Verification items for the finished model (mm, model axes). A direction names the side the tool comes from. Give positions to 0.01 mm unless a question says otherwise; leave off trailing zeros. Write each loop counter-clockwise with the first axis right and the second up, starting at its lowest first coordinate (ties: lowest second). Pieces come first, ordered by that corner, then holes.
from build123d import *

# Parameters (mm, degrees)
SKETCH_5_W          = 30.974653289
SKETCH_5_H          = 53.868777402
SKETCH_5_W_2        = 27.381586342
SKETCH_5_H_2        = 50.41539456
EXTRUDE_3_DEPTH     = 5
SKETCH_6_W          = 27.427442828
SKETCH_6_H          = 5
CUT_EXTRUDE_4_DEPTH = 4
SKETCH_8_W          = 6.119989238
SKETCH_8_H          = 1.581115617
CUT_EXTRUDE_6_DEPTH = 3
SKETCH_9_W          = 30.974653289
SKETCH_9_H          = 53.868777402
EXTRUDE_5_DEPTH     = 2
SKETCH_10_W         = 17.475002228
SKETCH_10_H         = 39.986467982
CUT_EXTRUDE_7_DEPTH = 1
FILLET_1_R          = 2
FILLET_2_R          = 2


with BuildPart() as part:
    # 草图5 → 凸台-拉伸3 (new body)
    with BuildSketch(Plane.XY.offset(17)):
        with Locations((52.154033433, -51.822040042)):
            Rectangle(SKETCH_5_W, SKETCH_5_H)
        with Locations((52.104679946, -51.967615846)):
            Rectangle(SKETCH_5_W_2, SKETCH_5_H_2, mode=Mode.SUBTRACT)
    extrude(amount=EXTRUDE_3_DEPTH)

    # 草图6 → 切除-拉伸4 (cut)
    with BuildSketch(Plane(origin=(0, -24.887651341, 0), x_dir=(1, 0, 0), z_dir=(0, 1, 0))):
        with Locations((52.127608189, -19.5)):
            Rectangle(SKETCH_6_W, SKETCH_6_H)
    extrude(amount=-CUT_EXTRUDE_4_DEPTH, mode=Mode.SUBTRACT)

    # 草图8 → 切除-拉伸6 (cut)
    with BuildSketch(Plane(origin=(0, 0, 17), x_dir=(-1, 0, 0), z_dir=(0, 0, -1))):
        with Locations((-52.130085605, -77.965870935)):
            Rectangle(SKETCH_8_W, SKETCH_8_H)
    extrude(amount=-CUT_EXTRUDE_6_DEPTH, mode=Mode.SUBTRACT)

    # 草图9 → 凸台-拉伸5 (add)
    with BuildSketch(Plane.XY.offset(22)):
        with Locations((52.154033433, -51.822040042)):
            Rectangle(SKETCH_9_W, SKETCH_9_H)
    extrude(amount=EXTRUDE_5_DEPTH)

    # 草图10 → 切除-拉伸7 (cut)
    with BuildSketch(Plane.XY.offset(24)):
        with Locations((52.039568352, -52.470675496)):
            Rectangle(SKETCH_10_W, SKETCH_10_H)
    extrude(amount=-CUT_EXTRUDE_7_DEPTH, mode=Mode.SUBTRACT)

    # 圆角1
    fillet_1_edges = [part.edges().sort_by_distance(p)[0] for p in [
        (67.641360077, -78.756428743, 20.5),
        (36.666706788, -78.756428743, 20.5),
        (36.666706788, -24.887651341, 20.5),
        (67.641360077, -24.887651341, 20.5),
    ]]
    fillet(fillet_1_edges, radius=FILLET_1_R)

    # 圆角2
    fillet_2_edges = [part.edges().sort_by_distance(p)[0] for p in [
        (43.302067238, -72.463909487, 23.5),
        (43.302067238, -32.477441505, 23.5),
        (60.777069466, -32.477441505, 23.5),
        (60.777069466, -72.463909487, 23.5),
    ]]
    fillet(fillet_2_edges, radius=FILLET_2_R)


solid = part.part
Item 1: Release check for a two-part mould opening along Y. For faces 5 (the face through (67.04, -78.186, 20.549)), 6 (the face through (65.841, -27, 20)), 7 (the face through (52, -52, 23)) record: released by +Y, released by -Y, zero draft, split by the parting line, or undercut.
Answer key:
face 5: released by -Y
face 6: zero draft
face 7: undercut
Item 2: Depth check by flat-ended pin: pin 1 (1 mm diameter, centred on x = 47, y = -42.5, fed in from +Z); pin 2 (1.7 mm diameter, centred on y = -78, z = 19, fed in from -X); pin 3 (2.5 mm diameter, centred on x = 54, z = 20, fed in from +Y). Enter the tip coordinate at first touch or a pass-through.
Answer key:
pin 1: stops at z = 23
pin 2: stops at x = 36.71
pin 3: stops at y = -77.18
Item 3: Sectioned sample at C-C on y = -63. Record the cut outline in (x, z), then the cut area to 3 significant figures.
Answer key:
outline: (36.67, 17) - (38.41, 17) - (38.41, 22) - (65.8, 22) - (65.8, 17) - (67.64, 17) - (67.64, 24) - (60.78, 24) - (60.78, 23) - (43.3, 23) - (43.3, 24) - (36.67, 24) - close
area: 62.4 mm2
Item 4: Scan lines: line 1 along X through (y, z) = (-54, 17.75); line 2 along Y through (x, z) = (50, 23.25); line 3 along X through (y, z) = (-57, 23.25). Record each from-to range of solid material in increasing order.
Answer key:
line 1: x = 36.67 to 38.41, 65.8 to 67.64
line 2: y = -78.76 to -72.46, -32.48 to -24.89
line 3: x = 36.67 to 43.3, 60.78 to 67.64
Item 5: Sectioned sample at D-D on x = 40. Record the cut outline in (y, z).
Answer key:
outline: (-78.76, 17) - (-77.18, 17) - (-77.18, 22) - (-24.89, 22) - (-24.89, 24) - (-78.76, 24) - close
Item 6: Sectioned sample at B-B on x = 46. Record the cut outline in (y, z), then the cut area to 3 significant figures.
Answer key:
outline: (-78.76, 17) - (-77.18, 17) - (-77.18, 22) - (-24.89, 22) - (-24.89, 24) - (-32.48, 24) - (-32.48, 23) - (-72.46, 23) - (-72.46, 24) - (-78.76, 24) - close
area: 75.7 mm2
Item 7: Sectioned sample at A-A on z = 17.75. Record the cut outline in (x, y).
Answer key:
outline: (36.67, -76.76) arc R2 ccw to (38.67, -78.76) - (49.07, -78.76) - (49.07, -77.18) - (38.41, -77.18) - (38.41, -24.9) arc R2 ccw to (36.67, -26.89) - close; (55.19, -78.76) - (65.64, -78.76) arc R2 ccw to (67.64, -76.76) - (67.64, -26.89) arc R2 ccw to (65.84, -24.9) - (65.84, -28.89) - (65.8, -28.89) - (65.8, -77.18) - (55.19, -77.18) - close
Item 8: Set-up check for faces 1 (the face through (60.18, -71.89, 23.49)), 2 (the face through (65.795, -53, 19)), 3 (the face through (38, -56, 17)), 4 (the face through (52, -78, 20)): record each of +Z, -Z, +X, -X, +Y, -Y from which the full face is reachable in a straight line by a thin tool's end or side.
Answer key:
face 1: +Z
face 2: -Z, +Y
face 3: -Z, +X, -X, +Y, -Y
face 4: -Z, +Y, -Y
